Source: CAD feature listing. Evaluate the final solid. Frame: model axes, mm. A direction names the side the tool comes from. Coordinates: 2 decimals unless noted, no trailing zeros. Loops run counter-clockwise (first coordinate to the right, second up) from the corner with the lowest first, then second, coordinate; pieces in that order, holes last.
Item 1: Section query A-A, the plane x = -1. Return the cut outline in (y, z), then the cut area to 3 significant figures.
Item 2: Pin query (flat end, axial travel): pin 1 Ø2 at (y, z) = (32.5, 56) entering from +X; pin 2 Ø2 at (y, z) = (24, 39.5) entering from +X; pin 3 Ø1.5 at (y, z) = (21.5, -34.5) entering from -X. Return the tip coordinate at first contact, or that it passes through.
Item 3: Section query B-B, the plane z = 61. Return the cut outline in (x, y).
Item 4: Section query D-D, the plane z = -15. Return the cut outline in (x, y), then the cut area to 3 significant figures.
Item 5: Pull-direction query (Z, two-part tool) for faces 4 (the cylindrical face through (-29.953, 25.756, 40.771)), 5 (the flat face through (0, 25, -65.718)), 6 (the flat face through (-27.57, 25.04, 60.71)); classes: +Z half, -Z half, draft (parallel to the pull), parting line (faces both ways), or undercut.
Item 6: Reachability of faces 1 (the flat face through (40.282, 25, -33)), 2 (the flat face through (-39.967, 25, -32)), 3 (the cylindrical face through (-58.316, 25.756, 31.669)) from +Z, -Z, +X, -X, +Y, -Y: full face, straight path, thin tool, end or side. Return the list, or none.
Item 7: Line query: probe 1 along Z at (x, y) = (0, 40); probe 2 along X at (y, z) = (44.5, -1); probe 3 along Z at (x, y) = (6, 14.5). Output: solid intervals per line, ascending.
Item 8: Section query C-C, the plane y = 41. Return the cut outline in (x, z), then the cut area to 3 significant figures.
```python
from build123d import *

# Parameters (mm, degrees)
F1_DEPTH = 50.8
F2_R     = 20.32
F3_R     = 25.4
F4_R     = 25.4
F5_R     = 31.402623
F6_DEPTH = 50.801


with BuildPart() as f1:
    # F0 (on Front) → F1 (new body)
    with BuildSketch(Plane.XZ):
        Polygon((-39.967455, -65.717764), (40.282056, -65.717764), (40.282056, 0), (76.221071, 33.392798), (0, 76.340705), (-75.760126, 33.392798), (-39.967455, 0), align=None)
    extrude(amount=-F1_DEPTH)

    # F2
    f2_edges = [f1.edges().sort_by_distance(p)[0] for p in [
        (0, 25.4, 76.340705),
    ]]
    fillet(f2_edges, radius=F2_R)

    # F3
    f3_edges = [f1.edges().sort_by_distance(p)[0] for p in [
        (76.221071, 25.4, 33.392798),
    ]]
    fillet(f3_edges, radius=F3_R)

    # F4
    f4_edges = [f1.edges().sort_by_distance(p)[0] for p in [
        (-75.760126, 25.4, 33.392798),
    ]]
    fillet(f4_edges, radius=F4_R)

    # F5 (on face) → F6 (cut, through all)
    with BuildSketch(Plane(origin=(0, 50.8, 0), x_dir=(-1, 0, 0), z_dir=(0, 1, 0))):
        with Locations((0, 31.338445)):
            Circle(F5_R)
    extrude(amount=-F6_DEPTH, mode=Mode.SUBTRACT)


solid = f1.part
```
Verdict:
1. outline: (0, -65.72) - (50.8, -65.72) - (50.8, -0.05) - (0, -0.05) - close; (0, 62.73) - (50.8, 62.73) - (50.8, 73.29) - (0, 73.29) - close
1. area: 3,870 mm2
2. pin 1: stops at x = 37.87
2. pin 2: stops at x = 56.74
2. pin 3: stops at x = -39.97
3. outline: (-27.06, 0) - (-10.31, 0) - (-10.31, 50.8) - (-27.06, 50.8) - close; (10.31, 0) - (27.23, 0) - (27.23, 50.8) - (10.31, 50.8) - close
4. outline: (-39.97, 0) - (40.28, 0) - (40.28, 50.8) - (-39.97, 50.8) - close
4. area: 4,080 mm2
5. face 4: undercut
5. face 5: -Z half
5. face 6: +Z half
6. face 1: -Z, +X, +Y, -Y
6. face 2: -Z, -X, +Y, -Y
6. face 3: -X, +Y, -Y
7. probe 1: z = -65.72 to -0.06, 62.74 to 73.32
7. probe 2: x = -39.97 to 40.28
7. probe 3: z = -65.72 to 0.51, 62.16 to 72.42
8. outline: (-50.46, 9.79) - (-39.97, 0) - (-39.97, -65.72) - (40.28, -65.72) - (40.28, 0) - (50.75, 9.73) arc R25.4 ccw to (45.93, 50.46) - (10.01, 70.7) arc R20.32 ccw to (-9.99, 70.68) - (-45.66, 50.46) arc R25.4 ccw to start; hole circle Ø62.81 at (0, 31.34)
8. area: 8,750 mm2
